Geometry: final body of the model. Coordinates: model frame, mm. Face numbers are marked on the shaded views. A direction names the side the tool comes from. Coordinates: 2 decimals unless noted, no trailing zeros. Order: outer loops, then holes, each group sorted by start corner. A loop starts at its lowest first (then second) coordinate and runs counter-clockwise, first axis right, second up. Notation, with made-up numbers: M 87,51.25 L 91,51.25 A18 cw 91,75.25 Z; hole C -9.75,-36 d6. An arc over 180 degrees is marked long. Use CSV: the item, a comma, the result in double quotes. Start each with the question number.
Q1. First-contact query: P1, Ø5, axis at x = 13, y = -3, coming from the -Z side; P2, Ø2, axis at x = 19, z = 17, coming from the -Y side; P3, Ø3, axis at x = 2.5, y = 9, coming from the +Z side; P4, Ø17.5, axis at y = 5, z = 5.5, coming from the +X side. Flat tips, straight axial feed; report the tip coordinate or a pass-through.
Q2. Ray query, probe 1 along Y at (x, z) = (2.95, 4.65); probe 2 along X at (y, z) = (-12.5, 11); probe 3 along Y at (x, z) = (6.75, 5). Return the intervals inside material, ascending.
Q3. Section query D-D, the plane x = 18.25. Output: boundary loops of the cut face in (y, z), and give its area (3 significant figures).
Q4. Section query A-A, the plane z = 16.65. Output: boundary loops of the cut face in (x, y).
Q5. Mould query, pull axis X, two halves, no side actions, for the marked faces 6, 7 and 8. Classes: +X half, -X half, draft (parallel to the pull), parting line (faces both ways), or undercut.
Q6. Section query C-C, the plane z = 20.5. Output: boundary loops of the cut face in (x, y), and give its area (3 significant figures).
Q7. Access query for the marked faces 1, 2, 3, 4 and 5. Directions: +Z, -Z, +X, -X, +Y, -Y. A direction counts if a zero-diameter tool reaches every point of the face in a straight line with its end or side. Return the directions, or none.
Q8. Section query B-B, the plane y = 15. Output: boundary loops of the cut face in (x, z), and give its area (3 significant figures).
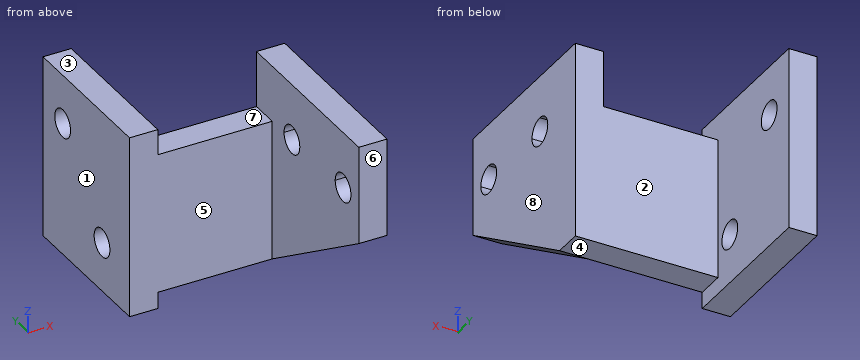
from build123d import *

# Parameters (mm, degrees)
BOSS_EXTRU_1_DEPTH      = 20
ESQUISSE3_W             = 4
ESQUISSE3_H             = 18
BOSS_EXTRU_2_DEPTH      = 20
ESQUISSE4_W             = 4
ESQUISSE4_H             = 18
BOSS_EXTRU_3_DEPTH      = 20
ESQUISSE5_W             = 17.65
ESQUISSE5_H             = 18
ESQUISSE5_W_2           = 16.35
ESQUISSE5_R             = 2
ENL_V_MAT_EXTRU_1_DEPTH = 20
ESQUISSE6_W             = 4
ESQUISSE6_H             = 26
BOSS_EXTRU_4_DEPTH      = 4
ESQUISSE7_R             = 2
ENL_V_MAT_EXTRU_2_DEPTH = 4
ESQUISSE8_R             = 2
ENL_V_MAT_EXTRU_3_DEPTH = 4
ESQUISSE9_W             = 4
ESQUISSE9_H             = 26
BOSS_EXTRU_5_DEPTH      = 8
ENL_V_MAT_EXTRU_5_DEPTH = 8


with BuildPart() as part:
    # Esquisse1 → Boss.-Extru.1 (new body)
    with BuildSketch(Plane.XY):
        Polygon((0, 16), (0, 0), (24.25, 0), (24.25, 2), (4, 2), (4, 16), align=None)
        Polygon((24.25, 0), (0, 0), (0, -2), (20.25, -2), (20.25, -24), (24.25, -24), align=None)
    extrude(amount=BOSS_EXTRU_1_DEPTH)

    # Esquisse3 → Boss.-Extru.2 (add)
    with BuildSketch(Plane(origin=(0, 0, 0), x_dir=(-1, 0, 0), z_dir=(0, 0, -1))):
        with Locations((-2, 7)):
            Rectangle(ESQUISSE3_W, ESQUISSE3_H)
    extrude(amount=BOSS_EXTRU_2_DEPTH)

    # Esquisse4 → Boss.-Extru.3 (add)
    with BuildSketch(Plane.XY.offset(20)):
        with Locations((2, 7)):
            Rectangle(ESQUISSE4_W, ESQUISSE4_H)
    extrude(amount=BOSS_EXTRU_3_DEPTH)

    # Esquisse5 → Enlèv. mat.-Extru.1 (cut)
    with BuildSketch(Plane.ZY):
        with Locations((-11.175, 7)):
            Rectangle(ESQUISSE5_W, ESQUISSE5_H)
        with Locations((31.825, 7)):
            Rectangle(ESQUISSE5_W_2, ESQUISSE5_H)
        with Locations((16.65, 15)):
            Circle(ESQUISSE5_R)
        with Locations((4.65, 5)):
            Circle(ESQUISSE5_R)
    extrude(amount=-ENL_V_MAT_EXTRU_1_DEPTH, mode=Mode.SUBTRACT)

    # Esquisse6 → Boss.-Extru.4 (add)
    with BuildSketch(Plane(origin=(0, 16, 0), x_dir=(1, 0, 0), z_dir=(0, 1, 0))):
        with Locations((2, -10.65)):
            Rectangle(ESQUISSE6_W, ESQUISSE6_H)
    extrude(amount=BOSS_EXTRU_4_DEPTH)

    # Esquisse7 → Enlèv. mat.-Extru.2 (cut)
    with BuildSketch(Plane.ZY):
        with Locations((16.65, 15)):
            Circle(ESQUISSE7_R)
    extrude(amount=-ENL_V_MAT_EXTRU_2_DEPTH, mode=Mode.SUBTRACT)

    # Esquisse8 → Enlèv. mat.-Extru.3 (cut)
    with BuildSketch(Plane.ZY.offset(-20.25)):
        with Locations((20, -7)):
            Circle(ESQUISSE8_R)
        with Locations((20, -20)):
            Circle(ESQUISSE8_R)
    extrude(amount=-ENL_V_MAT_EXTRU_3_DEPTH, mode=Mode.SUBTRACT)

    # Esquisse9 → Boss.-Extru.5 (add)
    with BuildSketch(Plane.XY.offset(20)):
        with Locations((22.25, -11)):
            Rectangle(ESQUISSE9_W, ESQUISSE9_H)
    extrude(amount=BOSS_EXTRU_5_DEPTH)

    # Esquisse11 → Enlèv. mat.-Extru.5 (cut)
    with BuildSketch(Plane.ZY.offset(-20.25)):
        with BuildLine():
            ThreePointArc((20, -9), (21.414213562, -8.414213562), (22, -7))
            ThreePointArc((22, -7), (21.414213562, -5.585786438), (20, -5))
            Line((20, -5), (20, -9))
        make_face()
        with BuildLine():
            Line((20, -9), (20, -5))
            ThreePointArc((20, -5), (18, -7), (20, -9))
        make_face()
        with BuildLine():
            ThreePointArc((20, -22), (21.414213562, -21.414213562), (22, -20))
            ThreePointArc((22, -20), (21.414213562, -18.585786438), (20, -18))
            Line((20, -18), (20, -22))
        make_face()
        with BuildLine():
            Line((20, -22), (20, -18))
            ThreePointArc((20, -18), (18, -20), (20, -22))
        make_face()
        Polygon((14, -24), (0, -2), (0, -24), align=None)
    extrude(amount=-ENL_V_MAT_EXTRU_5_DEPTH, mode=Mode.SUBTRACT)


solid = part.part
Responses:
1,P1,"stops at z = 0"
1,P2,"stops at y = -2"
1,P3,"stops at z = 23.65"
1,P4,"stops at x = 24.25"
2,probe 1,"y = -2 to 3, 7 to 20"
2,probe 2,"x = 20.25 to 24.25"
2,probe 3,"y = -2 to 2"
3,outline,"M -2,0 L 2,0 L 2,20 L -2,20 Z"
3,area,"80.0 mm²"
4,outline,"M 0,-2 L 20.25,-2 L 20.25,-24 L 24.25,-24 L 24.25,2 L 4,2 L 4,13 L 0,13 Z; M 0,17 L 4,17 L 4,20 L 0,20 Z"
5,face 6,"draft"
5,face 7,"undercut"
5,face 8,"+X half"
6,outline,"M 0,-2 L 4,-2 L 4,20 L 0,20 Z; M 20.25,-24 L 24.25,-24 L 24.25,-21.94 L 20.25,-21.94 Z; M 20.25,-18.06 L 24.25,-18.06 L 24.25,-8.94 L 20.25,-8.94 Z; M 20.25,-5.06 L 24.25,-5.06 L 24.25,2 L 20.25,2 Z"
6,area,"161 mm²"
7,face 1,"+Z, -Z, -X, +Y, -Y"
7,face 2,"+Z, -Z, +X, +Y"
7,face 3,"+Z, -X, +Y, -Y"
7,face 4,"-Z, +X, +Y, -Y"
7,face 5,"+Z, -Z, -X, -Y"
8,outline,"M 0,-2.35 L 4,-2.35 L 4,14.65 L 0,14.65 Z; M 0,18.65 L 4,18.65 L 4,23.65 L 0,23.65 Z"
8,area,"88.0 mm²"
